Can you work these out from the model? Positions are in its coordinate system, mm. Coordinates: 2 decimals unless noted, no trailing zeros. Loops run counter-clockwise (first coordinate to the right, second up) from the corner with the lowest first, then second, coordinate; pieces in that order, holes last. Notation, with made-up numbers: M 24.5,42.5 L 82.5,42.5 A23 ccw 82.5,57.5 Z; hole C -39,84 d1. An arc over 180 degrees is marked long. Return JSON: item names as keys, results as strings. Group by question number.
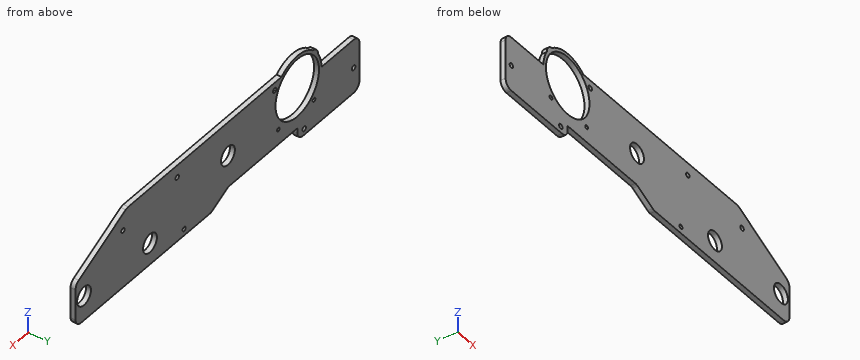
```python
from build123d import *

# Parameters (mm, degrees)
SKETCH1_W           = 210
SKETCH1_H           = 50
SKETCH1_R           = 1.211665018
SKETCH1_R_2         = 1.165617118
SKETCH1_R_3         = 1.5
SKETCH1_R_4         = 1.517273905
SKETCH1_R_5         = 1.335614121
SKETCH1_R_6         = 1.62438417
BOSS_EXTRUDE1_DEPTH = 3.175
SKETCH2_R           = 2
CUT_EXTRUDE1_DEPTH  = 10
SKETCH3_R           = 6
SKETCH3_R_2         = 0.586995366
CUT_EXTRUDE2_DEPTH  = 57.15
CUT_EXTRUDE7_DEPTH  = 10
FILLET3_R           = 5
SKETCH11_R          = 18.5
SKETCH11_R_2        = 2
BOSS_EXTRUDE4_DEPTH = 3.175
SKETCH12_R          = 21
BOSS_EXTRUDE5_DEPTH = 3.175
SKETCH13_R          = 18.85
CUT_EXTRUDE8_DEPTH  = 3.175
BOSS_EXTRUDE6_DEPTH = 3.175
FILLET4_R           = 5
SKETCH15_R          = 1.5
CUT_EXTRUDE9_DEPTH  = 10
SKETCH16_R          = 1.5
CUT_EXTRUDE10_DEPTH = 10
SKETCH17_R          = 1.5
CUT_EXTRUDE11_DEPTH = 10


with BuildPart() as part:
    # Sketch1 → Boss-Extrude1 (new body)
    with BuildSketch(Plane(origin=(0, 0, 0), x_dir=(1, 0, 0), z_dir=(0, 1, 0))):
        with Locations((105, -25)):
            Rectangle(SKETCH1_W, SKETCH1_H)
        with Locations(Location((3.489526233, -16.787661112, 0), (0, 0, 270))):
            Circle(SKETCH1_R, mode=Mode.SUBTRACT)
        with Locations(Location((34.37258772, -17.194005245, 0), (0, 0, 270))):
            Circle(SKETCH1_R_2, mode=Mode.SUBTRACT)
        with Locations(Location((37.520749958, -44.921198121, 0), (0, 0, 270))):
            Circle(SKETCH1_R_3, mode=Mode.SUBTRACT)
        with Locations(Location((168.975233936, -37.403209633, 0), (0, 0, 270))):
            Circle(SKETCH1_R_4, mode=Mode.SUBTRACT)
        with Locations(Location((116, -4.237214774, 0), (0, 0, 270))):
            Circle(SKETCH1_R_5, mode=Mode.SUBTRACT)
        with Locations(Location((12.257640281, -3.274812063, 0), (0, 0, 270))):
            Circle(SKETCH1_R_6, mode=Mode.SUBTRACT)
    extrude(amount=BOSS_EXTRUDE1_DEPTH)

    # Sketch2 → Cut-Extrude1 (cut)
    with BuildSketch(Plane(origin=(0, 3.175, 0), x_dir=(1, 0, 0), z_dir=(0, 1, 0))):
        with Locations(Location((10, -26, 0), (0, 0, 270))):
            Circle(SKETCH2_R)
        with Locations(Location((10, -42, 0), (0, 0, 270))):
            Circle(SKETCH2_R)
        with Locations(Location((26, -26, 0), (0, 0, 270))):
            Circle(SKETCH2_R)
        with Locations(Location((26, -42, 0), (0, 0, 270))):
            Circle(SKETCH2_R)
    extrude(amount=-CUT_EXTRUDE1_DEPTH, mode=Mode.SUBTRACT)

    # Sketch3 → Cut-Extrude2 (cut)
    with BuildSketch(Plane(origin=(0, 3.175, 0), x_dir=(1, 0, 0), z_dir=(0, 1, 0))):
        with Locations(Location((78.01026379, -28.1, 0), (0, 0, 270))):
            Circle(SKETCH3_R)
        with Locations(Location((145.531297368, -14, 0), (0, 0, 270))):
            Circle(SKETCH3_R)
        with Locations(Location((18, -34, 0), (0, 0, 270))):
            Circle(SKETCH3_R_2)
        with Locations(Location((202.646291021, -16, 0), (0, 0, 270))):
            Circle(SKETCH3_R)
    extrude(amount=-CUT_EXTRUDE2_DEPTH, mode=Mode.SUBTRACT)

    # Sketch10 → Cut-Extrude7 (cut)
    with BuildSketch(Plane(origin=(0, 3.175, 0), x_dir=(1, 0, 0), z_dir=(0, 1, 0))):
        Polygon((210, -27.859435908), (165.502877994, -50), (210, -50), align=None)
        Polygon((92.532613397, 0), (77.65477062, -7.402812063), (0, -7.402812063), (0, 0), align=None)
    extrude(amount=-CUT_EXTRUDE7_DEPTH, mode=Mode.SUBTRACT)

    # Fillet3
    fillet3_edges = [part.edges().sort_by_distance(p)[0] for p in [
        (210, 1.5875, 0),
        (0, 1.5875, 50),
        (92.532613397, 1.5875, 0),
        (210, 1.5875, 27.859435908),
        (165.502877994, 1.5875, 50),
        (77.65477062, 1.5875, 7.402812063),
        (0, 1.5875, 7.402812063),
    ]]
    fillet(fillet3_edges, radius=FILLET3_R)

    # Sketch11 → Boss-Extrude4 (add)
    with BuildSketch(Plane(origin=(0, 3.175, 0), x_dir=(1, 0, 0), z_dir=(0, 1, 0))):
        with Locations((18, -34)):
            Circle(SKETCH11_R)
        with Locations(Location((10, -26, 0), (0, 0, 270))):
            Circle(SKETCH11_R_2, mode=Mode.SUBTRACT)
        with Locations(Location((10, -42, 0), (0, 0, 270))):
            Circle(SKETCH11_R_2, mode=Mode.SUBTRACT)
        with Locations(Location((26, -26, 0), (0, 0, 270))):
            Circle(SKETCH11_R_2, mode=Mode.SUBTRACT)
        with Locations(Location((26, -42, 0), (0, 0, 270))):
            Circle(SKETCH11_R_2, mode=Mode.SUBTRACT)
    extrude(amount=-BOSS_EXTRUDE4_DEPTH)

    # Sketch12 → Boss-Extrude5 (add)
    with BuildSketch(Plane(origin=(0, 3.175, 0), x_dir=(1, 0, 0), z_dir=(0, 1, 0))):
        with Locations((18, -34)):
            Circle(SKETCH12_R)
    extrude(amount=-BOSS_EXTRUDE5_DEPTH)

    # Sketch13 → Cut-Extrude8 (cut)
    with BuildSketch(Plane(origin=(0, 3.175, 0), x_dir=(1, 0, 0), z_dir=(0, 1, 0))):
        with Locations(Location((18, -34, 0), (0, 0, 270))):
            Circle(SKETCH13_R)
    extrude(amount=-CUT_EXTRUDE8_DEPTH, mode=Mode.SUBTRACT)

    # Sketch14 → Boss-Extrude6 (add)
    with BuildSketch(Plane(origin=(0, 3.175, 0), x_dir=(1, 0, 0), z_dir=(0, 1, 0))):
        with BuildLine():
            Line((-35.83, -34.272812063), (-2.998227868, -34.272812063))
            ThreePointArc((-2.998227868, -34.272812063), (-2.272136238, -28.519079241), (0, -23.183346174))
            Line((0, -23.183346174), (0, -12.402812063))
            Line((0, -12.402812063), (0, -12.248529085))
            Line((0, -12.248529085), (0, 0.727187937))
            Line((0, 0.727187937), (-35.83, 0.727187937))
            Line((-35.83, 0.727187937), (-35.83, -34.272812063))
        make_face()
        with BuildLine():
            Line((0, 0.727187937), (0, -12.248529085))
            Line((0, -12.248529085), (0.002380891, -12.248529085))
            ThreePointArc((0.002380891, -12.248529085), (1.51944077, -8.813145304), (5, -7.402812063))
            Line((5, -7.402812063), (18, -7.402812063))
            Line((18, -7.402812063), (18, 0.727187937))
            Line((18, 0.727187937), (0, 0.727187937))
        make_face()
    extrude(amount=-BOSS_EXTRUDE6_DEPTH)

    # Fillet4
    fillet4_edges = [part.edges().sort_by_distance(p)[0] for p in [
        (-35.83, 1.5875, 34.272812063),
        (-35.83, 1.5875, -0.727187937),
        (18, 1.5875, -0.727187937),
    ]]
    fillet(fillet4_edges, radius=FILLET4_R)

    # Sketch15 → Cut-Extrude9 (cut)
    with BuildSketch(Plane(origin=(0, 3.175, 0), x_dir=(1, 0, 0), z_dir=(0, 1, 0))):
        with Locations(Location((122, -42.058139805, 0), (0, 0, 270))):
            Circle(SKETCH15_R)
    extrude(amount=-CUT_EXTRUDE9_DEPTH, mode=Mode.SUBTRACT)

    # Sketch16 → Cut-Extrude10 (cut)
    with BuildSketch(Plane(origin=(0, 3.175, 0), x_dir=(1, 0, 0), z_dir=(0, 1, 0))):
        with Locations(Location((12, -3.272812063, 0), (0, 0, 270))):
            Circle(SKETCH16_R)
    extrude(amount=-CUT_EXTRUDE10_DEPTH, mode=Mode.SUBTRACT)

    # Sketch17 → Cut-Extrude11 (cut)
    with BuildSketch(Plane(origin=(0, 3.175, 0), x_dir=(1, 0, 0), z_dir=(0, 1, 0))):
        with Locations(Location((-30.83, -15.772812063, 0), (0, 0, 270))):
            Circle(SKETCH17_R)
    extrude(amount=-CUT_EXTRUDE11_DEPTH, mode=Mode.SUBTRACT)


solid = part.part
```
1) If I drill on line 1 (X direction, y = 1.05, z = 41); line 2 (X direction, y = 1.2, z = 2); line 3 (Z direction, x = 116, y = 1.95), over which ranges is the centre line in solid material (lowest first)? Write a range as from..to.
2) For pin 1 (1.5 mm diameter, centred on y = 2, z = 45.5, fed in from -X); pin 2 (1.5 mm diameter, centred on x = 17, y = 2, fed in from +Z); pin 3 (1.8 mm diameter, centred on x = -30.83, z = 15.77, fed in from +Y); pin 4 (1 mm diameter, centred on y = 3, z = 47.5, fed in from +X), each with a flat end and sliding along its axis, tell me the tip position at first contact or that it passes through.
3) Suppose I cut it at C-C, the plane x = 100. List the corners of the cut face in (y, z) for me (3 decimals), then the cut area to 3 significant figures.
4) Suppose I cut it at A-A, the plane x = 67. List the corners of the cut face in (y, z) for me (3 decimals), then the cut area to 3 significant figures.
Returned:
{
 "1": {"line 1": "x = -1.8..0.5, 35.5..120.94, 123.06..183.59", "line 2": "x = -35.28..11.21, 12.79..17.45, 88.51..209", "line 3": "z = 0..2.9, 5.57..50"},
 "2": {"pin 1": "stops at x = -0.04", "pin 2": "stops at z = 55", "pin 3": "passes through", "pin 4": "stops at x = 171.53"},
 "3": {"outline": "M 0,0 L 3.175,0 L 3.175,50 L 0,50 Z", "area": "159 mm²"},
 "4": {"outline": "M 0,7.403 L 3.175,7.403 L 3.175,50 L 0,50 Z", "area": "135 mm²"}
}
